The listing builds one solid part. Answer for the finished solid, in the listing's coordinates (mm). Give positions to 0.01 mm unless a question says otherwise; leave off trailing zeros. Write each loop counter-clockwise with the first axis right and the second up, starting at its lowest first coordinate (ties: lowest second). Pieces come first, ordered by that corner, then holes. Notation, with made-up numbers: (5, -2) - (30, -2) arc R19 cw to (30, 25) - close; hole circle Ø4 at (71, -16). An arc over 180 degrees is marked (long way). Return JSON: item names as keys, results as strings.
Autodesk Inventor part; units mm, degrees
ref_plane "to_body_XY" through (0, 0, 0) normal (0, 0, 1) x (1, 0, 0)
ref_plane "to_body_YZ" through (0, 0, 0) normal (1, 0, 0) x (0, 1, 0)
ref_plane "to_body_ZX" through (0, 0, 0) normal (0, 1, 0) x (0, 0, 1)
sketch "_____1" plane through (0, 0, 0) normal (0, 0, 1) x (1, 0, 0)
  line L0 (50, 0) -> (-50, 0)
  line L1 (-4, 12) -> (-4, 4.5)
  line L2 (-4, 4.5) -> (-3.5, 4)
  line L3 (-3.5, 4) -> (3.5, 4)
  line L4 (3.5, 4) -> (4, 4.5)
  line L5 (4, 4.5) -> (4, 12)
  line L6 (4, 12) -> (3.5, 12.5)
  line L7 (3.5, 12.5) -> (-3.5, 12.5)
  line L8 (-3.5, 12.5) -> (-4, 12)
revolve "Revolution1" add sketch "_____1" angle 180 about axis through (50, 0, 0) along (-1, 0, 0)
sketch "_____2" plane through (0, 0, 0) normal (1, 0, 0) x (0, 0, -1)
  line L0 (-0.75, -25) -> (0.75, -25)
  line L1 (0.75, -25) -> (0.75, 25)
  line L2 (0.75, 25) -> (-0.75, 25)
  line L3 (-0.75, 25) -> (-0.75, -25)
extrude "Extrusion1" cut sketch "_____2" along normal mid plane 16
sketch "Sketch3" plane through (-3.5, 3.9291, -0.75) normal (0, 0, 1) x (1, 0, 0)
  point P0 (3.5, 4.0709)
hole "Hole1" at (0, 8, -0.75) direction (0, 0, -1) diameter 2.459 depth 12.5 countersink diameter 3 countersink angle 90
pattern_linear "Rectangular Pattern1" count 2 spacing 16 along (0, -1, 0) of "Hole1"
ref_plane "to_body_XY" through (0, 0, 0) normal (0, 0, 1) x (1, 0, 0)
ref_plane "to_body_YZ" through (0, 0, 0) normal (1, 0, 0) x (0, 1, 0)
ref_plane "to_body_ZX" through (0, 0, 0) normal (0, 1, 0) x (0, 0, 1)
properties part number "C-SCNPAW8-8_2"
Item 1: A cutting plane is placed at B-B on y = 0. Determine the outline of the cut face in (x, z), then the cut area to 3 significant figures.
Answer below:
{"outline": "(-4, -12) - (-3.5, -12.5) - (3.5, -12.5) - (4, -12) - (4, -4.5) - (3.5, -4) - (-3.5, -4) - (-4, -4.5) - close", "area": "67.5 mm²"}
Item 2: A cutting plane is placed at D-D on x = -1.75. Determine the outline of the cut face in (y, z), then the cut area to 3 significant figures.
Answer below:
{"outline": "(-12.48, -0.75) arc R12.5 ccw to (12.48, -0.75) - (3.93, -0.75) arc R4 cw to (-3.93, -0.75) - close", "area": "208 mm²"}
Item 3: A cutting plane is placed at C-C on z = -2. Give the number of separate pieces and of enclosed holes in the cut face, then the cut area to 3 significant figures.
Answer below:
{"separate pieces": "2", "enclosed holes": "2", "area": "131 mm²"}
Item 4: Flat-ended cylindrical pins translate along their axes: P1, Ø2, axis at x = 0, y = -8, coming from the -Z side; P2, Ø4, axis at x = -1, z = -9, coming from the +Y side. Find the tip coordinate at first contact, or state that the pin passes through.
Answer below:
{"P1": "passes through", "P2": "stops at y = 10.36"}
Item 5: The mould has two halves that part along X. Classify faces 1 (the face through (-2, -8, -0.75)), 2 (the face through (-0.05, -6.77, -5.83)), 3 (the face through (4, 0, -6)), 4 (the face through (-3.64, 0.08, -4.14)): +X half, -X half, draft (parallel to the pull), parting line (faces both ways), or undercut.
Answer below:
{"face 1": "draft", "face 2": "undercut", "face 3": "+X half", "face 4": "-X half"}
Item 6: Consider L1, parallel to X at y = -8, z = -4; L2, parallel to Y at x = 0, z = -7.75; L3, parallel to Y at x = 0, z = -4.25. Determine where each line is inside the solid, lowest interval first.
Answer below:
{"L1": "x = -4 to -1.23, 1.23 to 4", "L2": "y = -9.81 to -9.23, -6.77 to 6.77, 9.23 to 9.81", "L3": "y = -11.76 to -9.23, -6.77 to 6.77, 9.23 to 11.76"}
Item 7: A cutting plane is placed at A-A on x = 0. Determine the outline of the cut face in (y, z).
Answer below:
{"outline": "(-12.48, -0.75) arc R12.5 ccw to (-9.23, -8.43) - (-9.23, -1.02) - (-9.5, -0.75) - close; (-6.77, -10.51) arc R12.5 ccw to (6.77, -10.51) - (6.77, -1.02) - (6.5, -0.75) - (3.93, -0.75) arc R4 cw to (-3.93, -0.75) - (-6.5, -0.75) - (-6.77, -1.02) - close; (9.23, -8.43) arc R12.5 ccw to (12.48, -0.75) - (9.5, -0.75) - (9.23, -1.02) - close"}
